Verification items for the finished model (mm, model axes). Face numbers are marked on the shaded views. Coordinates: 2 decimals unless noted, no trailing zeros. Loops run counter-clockwise (first coordinate to the right, second up) from the corner with the lowest first, then second, coordinate; pieces in that order, holes last. Notation, with made-up numbers: (70.5, 69) -> (114.5, 69) arc R36 cw to (114.5, 108) -> close; hole circle Ø2 at (23.25, 83.25). An arc over 180 degrees is marked (long way). Answer as a JSON object with one key per item and string values. Group by question number.
Q1. Cross-section at A-A on y = 17. Give the number of separate pieces and of enclosed holes in the cut face, and give its area (3 significant figures).
Q2. Scan lines: L1, parallel to Z at x = 40.5, y = 17.5; L2, parallel to X at y = 23, z = 3 (3 decimals); L3, parallel to X at y = 19, z = 5. Record each from-to range of solid material in increasing order.
Q3. Release check for a two-part mould opening along Z. For the marked faces 1 and 2 record: released by +Z, released by -Z, zero draft, split by the parting line, or undercut.
Q4. Gauge pin test, flat ends, axial feed: pin 1 Ø11 at (x, y) = (56.5, 9.5) entering from -Z; pin 2 Ø5 at (x, z) = (107.5, 43) entering from +Y; pin 3 Ø14.5 at (x, z) = (55, -46.5) entering from +Y (3 decimals). Record the tip position at first contact, or that the pin passes through.
Q5. Cross-section at C-C on z = -49. Record the boundary of the cut face in (x, y) (3 decimals).
```python
from build123d import *

# Parameters (mm, degrees)
BOSS_EXTRUDE1_DEPTH = 1
BOSS_EXTRUDE2_DEPTH = 25.4
SKETCH4_R           = 14.351
CUT_EXTRUDE1_DEPTH  = 25.4
SKETCH4_4_R         = 19.177
CUT_EXTRUDE2_DEPTH  = 22.225
LPATTERN1_COUNT     = 3
LPATTERN1_PITCH     = 78
SPLIT3_START        = -1
SPLIT3_DEPTH        = 27.4


# Read off the part's stored shape, not the designer's step: Split3
with BuildPart() as part:
    # Sketch1 → Boss-Extrude1 (new, symmetric)
    with BuildSketch(Plane(origin=(0, 0, 0), x_dir=(1, 0, 0), z_dir=(0, 1, 0))):
        Polygon((118, 0), (-118, 0), (-118, -67.135), (118, -75), align=None)
        Polygon((-118, 67.135), (-118, 0), (118, 0), (118, 75), align=None)
    extrude(amount=BOSS_EXTRUDE1_DEPTH, both=True)

    # Sketch3 → Boss-Extrude2 (add)
    with BuildSketch(Plane(origin=(0, 1, 0), x_dir=(1, 0, 0), z_dir=(0, 1, 0))):
        Polygon((-84.001477372, 20.6375), (-73.002954744, 39.6875), (-84.001477372, 58.7375), (-105.998522628, 58.7375), (-116.997045256, 39.6875), (-105.998522628, 20.6375), align=None)
        Polygon((-38.632571531, 19.84375), (-49.631094159, 0.79375), (-71.628139415, 0.79375), (-82.626662043, 19.84375), (-71.628139415, 38.89375), (-49.631094159, 38.89375), align=None)
        Polygon((-84.001477372, -19.05), (-73.002954744, 0), (-84.001477372, 19.05), (-105.998522628, 19.05), (-116.997045256, 0), (-105.998522628, -19.05), align=None)
        Polygon((-105.998522628, -58.7375), (-84.001477372, -58.7375), (-73.002954744, -39.6875), (-84.001477372, -20.6375), (-105.998522628, -20.6375), (-116.997045256, -39.6875), align=None)
        Polygon((-71.628139415, -38.89375), (-49.631094159, -38.89375), (-38.632571531, -19.84375), (-49.631094159, -0.79375), (-71.628139415, -0.79375), (-82.626662043, -19.84375), align=None)
    boss_extrude2 = extrude(amount=BOSS_EXTRUDE2_DEPTH)

    # Sketch4 → Cut-Extrude1 (cut)
    with BuildSketch(Plane(origin=(0, 26.4, 0), x_dir=(1, 0, 0), z_dir=(0, 1, 0))):
        with Locations(Location((-95, 0, 0), (0, 0, 270))):
            Circle(SKETCH4_R)
        with Locations(Location((-95, -39.6875, 0), (0, 0, 270))):
            Circle(SKETCH4_R)
        with Locations(Location((-95, 39.6875, 0), (0, 0, 90))):
            Circle(SKETCH4_R)
        with Locations(Location((-60.629616787, 19.84375, 0), (0, 0, 270))):
            Circle(SKETCH4_R)
        with Locations(Location((-60.629616787, -19.84375, 0), (0, 0, 90))):
            Circle(SKETCH4_R)
    cut_extrude1 = extrude(amount=-CUT_EXTRUDE1_DEPTH, mode=Mode.SUBTRACT)

    # Sketch4<4> → Cut-Extrude2 (cut)
    with BuildSketch(Plane(origin=(0, 26.4, 0), x_dir=(1, 0, 0), z_dir=(0, 1, 0))):
        with Locations((-95, 0)):
            Circle(SKETCH4_4_R)
        with Locations((-95, -39.6875)):
            Circle(SKETCH4_4_R)
        with Locations((-95, 39.6875)):
            Circle(SKETCH4_4_R)
        with Locations((-60.629616787, 19.84375)):
            Circle(SKETCH4_4_R)
        with Locations((-60.629616787, -19.84375)):
            Circle(SKETCH4_4_R)
    cut_extrude2 = extrude(amount=-CUT_EXTRUDE2_DEPTH, mode=Mode.SUBTRACT)

    # LPattern1: Boss-Extrude2, Cut-Extrude1, Cut-Extrude2 ×3
    with Locations(*[(i * LPATTERN1_PITCH, 0, 0) for i in range(1, LPATTERN1_COUNT)]):
        add(boss_extrude2)
        add(cut_extrude1, mode=Mode.SUBTRACT)
        add(cut_extrude2, mode=Mode.SUBTRACT)

    # Split3 outline → Split3 (cut)
    with BuildSketch(Plane(origin=(0, 0, 0), x_dir=(1, 0, 0), z_dir=(0, 1, 0)).offset(SPLIT3_START)):
        Polygon((15.04996756, -71.5690593), (44.913588808, -19.84375), (33.456794404, 0), (44.913588808, 19.84375), (15.04996756, 71.5690593), (-118, 67.135), (-118, -67.135), align=None)
    extrude(amount=SPLIT3_DEPTH, mode=Mode.SUBTRACT)


solid = part.part
```
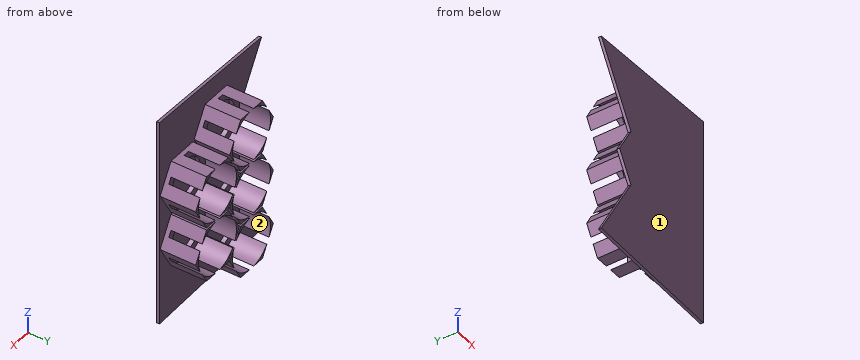
Computed values:
{
 "1": {"separate pieces": "30", "enclosed holes": "0", "area": "520 mm²"},
 "2": {"L1": "z = -42.28 to -37.09, -2.59 to 2.59, 37.09 to 42.28", "L2": "x = 40.735 to 42.059, 79.941 to 81.265, 83.098 to 86.203, 104.538 to 107.643", "L3": "x = 41.89 to 42.49, 79.51 to 80.11, 81.94 to 83.23, 107.51 to 108.8"},
 "3": {"face 1": "zero draft", "face 2": "undercut"},
 "4": {"pin 1": "stops at z = -58.74", "pin 2": "stops at y = 1", "pin 3": "stops at y = 4.175"},
 "5": {"outline": "(28.08, -1) -> (118, -1) -> (118, 1) -> (77.62, 1) -> (77.62, 4.175) -> (71.919, 4.175) -> (71.919, 1) -> (50.081, 1) -> (50.081, 4.175) -> (44.38, 4.175) -> (44.38, 1) -> (28.08, 1) -> close"}
}
